Could you check a few things on this model? Use its own coordinates, in mm. A direction names the side the tool comes from. Give positions to 0.01 mm unless a question says otherwise; leave off trailing zeros. Order: outer loops, then holes, each group sorted by start corner. A loop starts at its lowest first (then second) coordinate and runs counter-clockwise, first axis right, second up. Notation, with made-up numbers: (3, -19) -> (49, -19) arc R26 ccw to (49, 15) -> close; hole circle Ø11 at (31.25, -10). An arc over 180 degrees is marked (long way). One line per item, written item: value.
```python
from build123d import *

# Parameters (mm, degrees)
SKETCH1_R           = 2.3
BOSS_EXTRUDE1_DEPTH = 12.065
SKETCH5_R           = 1.5
SKETCH5_W           = 12.5
SKETCH5_H           = 2.065
CUT_EXTRUDE3_DEPTH  = 28.813022579
SKETCH6_W           = 18
SKETCH6_H           = 10
CUT_EXTRUDE5_DEPTH  = 32.07352933
SKETCH9_W           = 20
SKETCH9_H           = 1
CUT_EXTRUDE8_DEPTH  = 12.5
BOSS_EXTRUDE2_START = -24.13
SKETCH7_R           = 2.3
BOSS_EXTRUDE2_DEPTH = 24.13
SKETCH8_W           = 12.5
SKETCH8_H           = 1
CUT_EXTRUDE6_DEPTH  = 1
FILLET3_R           = 2
CUT_EXTRUDE9_DEPTH  = 14.5


with BuildPart() as part:
    # Sketch1 → Boss-Extrude1 (new, symmetric)
    with BuildSketch(Plane.XY):
        Polygon((22, -6), (0, -6), (-6, -6), (-6, 6), (0, 6), (11, 6), (22, -0.350852961), align=None)
        with Locations(Location((0, 0, 0), (0, 0, 180))):
            Circle(SKETCH1_R, mode=Mode.SUBTRACT)
    extrude(amount=BOSS_EXTRUDE1_DEPTH, both=True)

    # Sketch5 → Cut-Extrude3 (cut, through all)
    with BuildSketch(Plane(origin=(0, 6, 0), x_dir=(1, 0, 0), z_dir=(0, 1, 0))):
        with Locations(Location((18, 6.0325, 0), (0, 0, 270))):
            Circle(SKETCH5_R)
        with Locations(Location((18, 0, 0), (0, 0, 270))):
            Circle(SKETCH5_R)
        with Locations(Location((18, -6.0325, 0), (0, 0, 270))):
            Circle(SKETCH5_R)
        with Locations(Location((10, 0, 0), (0, 0, 270))):
            Circle(SKETCH5_R)
        with Locations((0.25, -11.0325)):
            Rectangle(SKETCH5_W, SKETCH5_H)
        with Locations((0.25, 11.0325)):
            Rectangle(SKETCH5_W, SKETCH5_H)
    extrude(amount=-CUT_EXTRUDE3_DEPTH, mode=Mode.SUBTRACT)

    # Sketch6 → Cut-Extrude5 (cut, through all)
    with BuildSketch(Plane.ZY.offset(6)):
        with Locations((0, 1)):
            Rectangle(SKETCH6_W, SKETCH6_H)
    extrude(amount=-CUT_EXTRUDE5_DEPTH, mode=Mode.SUBTRACT)

    # Sketch9 → Cut-Extrude8 (cut)
    with BuildSketch(Plane.ZY.offset(6)):
        with Locations((0, -5.5)):
            Rectangle(SKETCH9_W, SKETCH9_H)
    extrude(amount=-CUT_EXTRUDE8_DEPTH, mode=Mode.SUBTRACT)

    # Sketch7 → Boss-Extrude2 (add)
    with BuildSketch(Plane.XY.offset(12.065).offset(BOSS_EXTRUDE2_START)):
        Circle(SKETCH7_R)
    extrude(amount=BOSS_EXTRUDE2_DEPTH)

    # Sketch8 → Cut-Extrude6 (cut)
    with BuildSketch(Plane(origin=(0, 6, 0), x_dir=(1, 0, 0), z_dir=(0, 1, 0))):
        with Locations((0.25, -9.5)):
            Rectangle(SKETCH8_W, SKETCH8_H)
        with Locations((0.25, 9.5)):
            Rectangle(SKETCH8_W, SKETCH8_H)
    extrude(amount=-CUT_EXTRUDE6_DEPTH, mode=Mode.SUBTRACT)

    # Fillet3
    # the kernel refuses this fillet: 2 mm, written as the material it takes off along each edge
    with BuildSketch(Plane(origin=(-6, -5, 15), x_dir=(1, 0, 0), z_dir=(0, 0, -1))) as fillet3_piece_1:
        with BuildLine():
            CenterArc((FILLET3_R, -FILLET3_R), FILLET3_R, 90, 90)
            Line((0, -FILLET3_R), (0, 0))
            Line((0, 0), (FILLET3_R, 0))
        make_face()
    extrude(amount=30, mode=Mode.SUBTRACT)
    with BuildSketch(Plane(origin=(-6, 5, -15), x_dir=(1, 0, 0), z_dir=(0, 0, 1)), Plane(origin=(-6, 5, 4), x_dir=(1, 0, 0), z_dir=(0, 0, 1))) as fillet3_piece_2:
        with BuildLine():
            CenterArc((FILLET3_R, -FILLET3_R), FILLET3_R, 90, 90)
            Line((0, -FILLET3_R), (0, 0))
            Line((0, 0), (FILLET3_R, 0))
        make_face()
    extrude(amount=11, mode=Mode.SUBTRACT)

    # Sketch10 → Cut-Extrude9 (cut)
    with BuildSketch(Plane(origin=(22, 0, 0), x_dir=(0, 0, -1), z_dir=(1, 0, 0))):
        Polygon((-9, -4), (-9, 6), (-11.065, 6), (-11.065, -4), (-11.065, -5), (11.065, -5), (11.065, -4), (11.065, 6), (9, 6), (9, -4), align=None)
    extrude(amount=-CUT_EXTRUDE9_DEPTH, mode=Mode.SUBTRACT)


solid = part.part
```
1) Suppose I cut it at D-D, the plane z = 2.5. Write out the boundary of the cut face in (x, y).
Answer below:
outline: (-5.73, -4) arc R2 ccw to (-4, -5) -> (6.5, -5) -> (6.5, -6) -> (22, -6) -> (22, -5) -> (7.5, -5) -> (7.5, -4) -> close; circle Ø4.6 at (0, 0)
2) For P1, Ø3, axis at x = -3, y = 4, coming from the -Z side; P2, Ø5, axis at x = 0, z = 5, coming from the +Y side; P3, Ø4, axis at y = -1, z = -0.5, coming from the -X side, each with a flat end and sliding along its axis, tell me the tip position at first contact or that it passes through.
Answer below:
P1: stops at z = -10
P2: stops at y = 2.3
P3: stops at x = -2.3
3) If I drill on line 1 along Z through (x, y) = (-5, -0.25); line 2 along X through (y, z) = (-5.7, 0); line 3 along Z through (x, y) = (12.5, 1) (3 decimals), over which ranges is the centre line in solid material (lowest first)?
Answer below:
line 1: z = -10 to -9, 9 to 10
line 2: x = 6.5 to 8.5, 11.5 to 16.5, 19.5 to 22
line 3: z = -12.065 to -11.065, 11.065 to 12.065
4) Suppose I cut it at B-B, the plane z = 0. Write out the boundary of the cut face in (x, y).
Answer below:
outline: (-5.73, -4) arc R2 ccw to (-4, -5) -> (6.5, -5) -> (6.5, -6) -> (8.5, -6) -> (8.5, -5) -> (7.5, -5) -> (7.5, -4) -> close; circle Ø4.6 at (0, 0); (11.5, -6) -> (16.5, -6) -> (16.5, -5) -> (11.5, -5) -> close; (19.5, -6) -> (22, -6) -> (22, -5) -> (19.5, -5) -> close
5) Suppose I cut it at C-C, the plane y = 4.5. Write out the boundary of the cut face in (x, z) (3 decimals).
Answer below:
outline: (-5.323, -10) -> (6.5, -10) -> (6.5, -12.065) -> (13.598, -12.065) -> (13.598, -11.065) -> (7.5, -11.065) -> (7.5, -9) -> (-5.323, -9) -> close; (-5.323, 9) -> (7.5, 9) -> (7.5, 11.065) -> (13.598, 11.065) -> (13.598, 12.065) -> (6.5, 12.065) -> (6.5, 10) -> (-5.323, 10) -> close
6) For faces 5 (the flat face through (1.2, 5, -9.5)), 6 (the flat face through (7.5, -4.4, 1.7)), 7 (the flat face through (1, -5, 0)), 8 (the cylindrical face through (-1.825, -1.4, -0.126)), which set-ups out of +Z, -Z, +X, -X, +Y, -Y let a thin tool reach every point of the face, with its end or its side?
Answer below:
face 5: +Z, -Z, -X, +Y
face 6: +X, +Y
face 7: +Z, -Z, -X, -Y
face 8: none
7) Suppose I cut it at A-A, the plane x = 10. Write out the boundary of the cut face in (y, z) (3 decimals).
Answer below:
outline: (-6, -12.065) -> (6, -12.065) -> (6, -11.065) -> (-5, -11.065) -> (-5, -1.5) -> (-6, -1.5) -> close; (-6, 1.5) -> (-5, 1.5) -> (-5, 11.065) -> (6, 11.065) -> (6, 12.065) -> (-6, 12.065) -> close
8) We'd pull the mould along Z, two halves only. Please class faces 1 (the flat face through (2, 2, 9)), 2 (the flat face through (13, -1, 11.065)), 3 (the flat face through (2, -2, -10)), 4 (the flat face through (-6, 0, 9.5)): +Z half, -Z half, draft (parallel to the pull), parting line (faces both ways), or undercut.
Answer below:
face 1: undercut
face 2: undercut
face 3: -Z half
face 4: draft
